```python
from build123d import *

# Parameters (mm, degrees)
PAD015_DEPTH                        = 3
SKETCH054_R                         = 1.65
POCKET018_DEPTH                     = 358.938883
POCKET018_DEPTH_BACK                = 361.938883
BODY001003005003004_PLACEMENT_ANGLE = 60
CLONE005_PLACEMENT_ANGLE            = 19


with BuildPart() as part:
    # Sketch053 → Pad015 (new body)
    with BuildSketch(Plane.XY):
        with BuildLine():
            ThreePointArc((152.005097, 113.785532), (84.992984, 169.790723), (0, 189.875477))
            Line((0, 189.875477), (0, 196.875477))
            ThreePointArc((157.608957, 117.98038), (88.126358, 176.050273), (0, 196.875477))
            ThreePointArc((152.005097, 113.785532), (156.904451, 113.081026), (157.608957, 117.98038))
        make_face()
    pad015 = extrude(amount=PAD015_DEPTH)

    # Sketch054 → Pocket018 (cut, two sides)
    with BuildSketch(Plane.XY) as pocket018_sk:
        with Locations((150.82443, 121.020933)):
            Circle(SKETCH054_R)
        with BuildLine():
            ThreePointArc((0, 191.725477), (1.65, 193.375477), (0, 195.025477))
            Line((0, 191.725477), (0, 195.025477))
        make_face()
    pocket018 = extrude(amount=-POCKET018_DEPTH, mode=Mode.SUBTRACT) + extrude(pocket018_sk.sketch, amount=POCKET018_DEPTH_BACK, mode=Mode.SUBTRACT)

    # Mirrored020: Pad015, Pocket018 across Sketch053 V_Axis
    add(pad015.mirror(Plane(origin=(0, 0, 0), x_dir=(0, 0, 1), z_dir=(1, 0, 0))))
    add(pocket018.mirror(Plane(origin=(0, 0, 0), x_dir=(0, 0, 1), z_dir=(1, 0, 0))), mode=Mode.SUBTRACT)


with BuildPart() as part_1:
    # Body001003005003004 placement: moved
    add(part.part.rotate(Axis((0, 0, 0), (0, 0, 1)), BODY001003005003004_PLACEMENT_ANGLE))


with BuildPart() as part_2:
    # Clone005 placement: moved
    add(part_1.part.moved(Location((1038, 469, 0))).rotate(Axis((1038, 469, 0), (0, 0, -1)), CLONE005_PLACEMENT_ANGLE))


solid = part_2.part
```
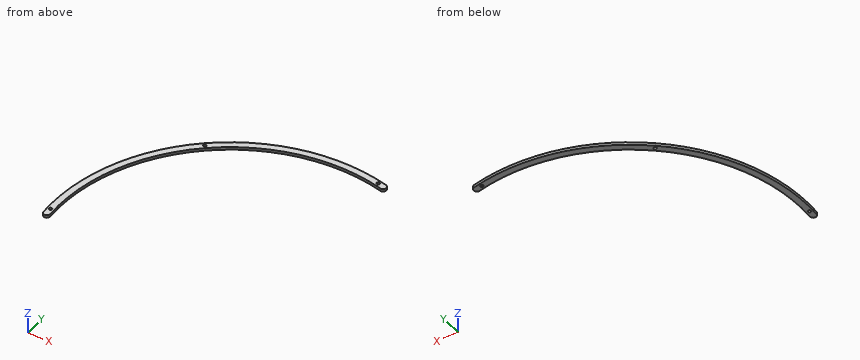
The model under review builds one solid part; all positions refer to its coordinate system, in mm. Coordinates: 2 decimals unless noted, no trailing zeros. Write each loop counter-clockwise with the first axis right and the second up, starting at its lowest first coordinate (ties: lowest second). Pieces come first, ordered by that corner, then holes. Notation, with made-up numbers: (-32, 47) - (11, 47) arc R32 ccw to (11, 83) - close; hole circle Ø9 at (28, 24). An arc over 180 degrees is marked (long way). Answer in a Markdown table with one row per item. Add a question column.
Q1. Consider section B-B on y = 639.5. Give the boundary of the cut face in (x, z), then the cut area to 3 significant figures.
Q2. Consider section A-A on z = 0.75. Give the boundary of the cut face in (x, y), then the cut area to 3 significant figures.
Q3. To check wall thickness, follow line 1 along Y through (x, z) = (1071, 2.1); line 2 along Y through (x, z) = (933, 2.85); line 3 along Y through (x, z) = (1027.5, 1.95). State the ranges of each line that lie inside material, in increasing order. Write a range as from..to.
Q4. Consider section C-C on x = 958.5. Give the boundary of the cut face in (y, z).
Q5. Clearance check with flat-ended pins moving along their axes: pin 1 (1 mm diameter, centred on x = 931, z = 2, fed in from -Y); pin 2 (4.5 mm diameter, centred on x = 1072.43, y = 659.29, fed in from -Z). State where each tip first meets the part, or that it passes through.
Answers below:
| question | item | result |
|---|---|---|
| 1 | outline | (939.56, 0) - (954.44, 0) - (954.44, 3) - (939.56, 3) - close |
| 1 | area | 44.6 mm² |
| 2 | outline | (841.65, 454.64) arc R3.5 ccw to (848.63, 455.15) arc R189.88 cw to (913.43, 612.3) arc R189.88 cw to (1078.07, 654.6) arc R3.5 ccw to (1079.55, 661.44) arc R196.88 ccw to (908.84, 617.58) arc R196.88 ccw to start; hole circle Ø3.3 at (844.77, 461.39); hole circle Ø3.3 at (911.13, 614.94); hole circle Ø3.3 at (1072.43, 659.29) |
| 2 | area | 2,530 mm² |
| 3 | line 1 | 655.99..658.47, 660.11..663.09 |
| 3 | line 2 | 627.2..635.54 |
| 3 | line 3 | 658.58..665.6 |
| 4 | outline | (641.43, 0) - (649.11, 0) - (649.11, 3) - (641.43, 3) - close |
| 5 | pin 1 | y = 625.51 |
| 5 | pin 2 | z = 0 |
